Build history of the part. All positions in model axes, mm. Face numbers are marked on the shaded views. A direction names the side the tool comes from. Round coordinates to 2 decimals unless told otherwise and drop trailing zeros. Write each loop counter-clockwise with the first axis right and the second up, starting at its lowest first coordinate (ties: lowest second). Pieces come first, ordered by that corner, then holes.
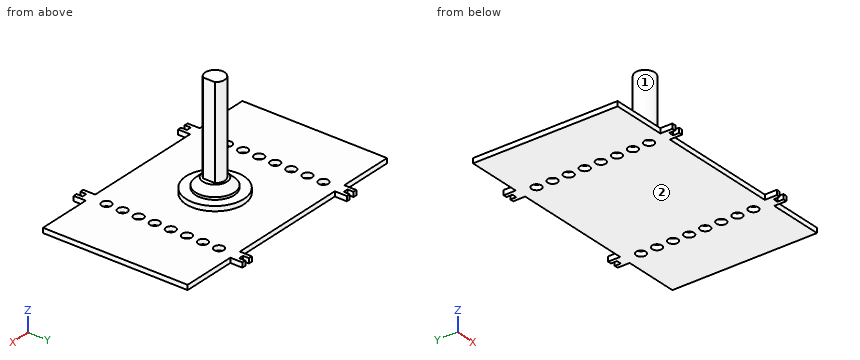
from build123d import *

# Parameters (mm, degrees)
SKETCH_R     = 2
PAD_DEPTH    = 2
SKETCH001_R  = 4
PAD001_DEPTH = 46
SKETCH002_R  = 8
PAD002_DEPTH = 8
SKETCH003_R  = 12
PAD003_DEPTH = 4
POCKET_DEPTH = 38
CHAMFER_SIZE = 3


with BuildPart() as part:
    # Sketch → Pad (new body)
    with BuildSketch(Plane.XY):
        Polygon((105, 0), (105, 60), (82.5, 60), (82.5, 65), (81, 65), (81, 62.5), (80, 62.5), (79, 62.5), (79, 65), (77.5, 65), (77.5, 60), (27.5, 60), (27.5, 65), (26, 65), (26, 62.5), (25, 62.5), (24, 62.5), (24, 65), (22.5, 65), (22.5, 60), (0, 60), (0, 0), (22.5, 0), (22.5, -5), (24, -5), (24, -2.5), (25, -2.5), (26, -2.5), (26, -5), (27.5, -5), (27.5, 0), (77.5, 0), (77.5, -5), (79, -5), (79, -2.5), (80, -2.5), (81, -2.5), (81, -5), (82.5, -5), (82.5, 0), align=None)
        with Locations((25, 46.666667)):
            Circle(SKETCH_R, mode=Mode.SUBTRACT)
        with Locations((25, 40)):
            Circle(SKETCH_R, mode=Mode.SUBTRACT)
        with Locations((25, 33.333333)):
            Circle(SKETCH_R, mode=Mode.SUBTRACT)
        with Locations((25, 26.666667)):
            Circle(SKETCH_R, mode=Mode.SUBTRACT)
        with Locations((25, 20)):
            Circle(SKETCH_R, mode=Mode.SUBTRACT)
        with Locations((25, 13.333333)):
            Circle(SKETCH_R, mode=Mode.SUBTRACT)
        with Locations((25, 6.666667)):
            Circle(SKETCH_R, mode=Mode.SUBTRACT)
        with Locations((80, 6.666667)):
            Circle(SKETCH_R, mode=Mode.SUBTRACT)
        with Locations((80, 13.333333)):
            Circle(SKETCH_R, mode=Mode.SUBTRACT)
        with Locations((80, 20)):
            Circle(SKETCH_R, mode=Mode.SUBTRACT)
        with Locations((80, 26.666667)):
            Circle(SKETCH_R, mode=Mode.SUBTRACT)
        with Locations((80, 33.333333)):
            Circle(SKETCH_R, mode=Mode.SUBTRACT)
        with Locations((80, 46.666667)):
            Circle(SKETCH_R, mode=Mode.SUBTRACT)
        with Locations((80, 40)):
            Circle(SKETCH_R, mode=Mode.SUBTRACT)
        with Locations((25, 53.333333)):
            Circle(SKETCH_R, mode=Mode.SUBTRACT)
        with Locations((80, 53.333333)):
            Circle(SKETCH_R, mode=Mode.SUBTRACT)
    extrude(amount=PAD_DEPTH)

    # Sketch001 → Pad001 (join)
    with BuildSketch(Plane.XY):
        with Locations((52.5, 30)):
            Circle(SKETCH001_R)
    extrude(amount=PAD001_DEPTH)

    # Sketch002 → Pad002 (join)
    with BuildSketch(Plane.XY):
        with Locations((52.5, 30)):
            Circle(SKETCH002_R)
    extrude(amount=PAD002_DEPTH)

    # Sketch003 → Pad003 (join)
    with BuildSketch(Plane.XY):
        with Locations((52.5, 30)):
            Circle(SKETCH003_R)
    extrude(amount=PAD003_DEPTH)

    # Sketch004 → Pocket (cut)
    with BuildSketch(Plane.XY.offset(46)):
        with BuildLine():
            Line((55.622499, 32.5), (55.622499, 27.5))
            ThreePointArc((55.622499, 27.5), (56.5, 30), (55.622499, 32.5))
        make_face()
    extrude(amount=-POCKET_DEPTH, mode=Mode.SUBTRACT)

    # Chamfer
    chamfer_edges = [part.edges().sort_by_distance(p)[0] for p in [
        (44.5, 30, 8),
    ]]
    chamfer(chamfer_edges, length=CHAMFER_SIZE)


solid = part.part
1) Which spindle directions (+Z, -Z, +X, -X, +Y, -Y) get a long thin tool onto all of the face, cutting with end or side? Do the marked faces 1 and 2. Say none if no direction does.
Results:
face 1: +Z
face 2: -Z, +X, -X, +Y, -Y
2) Slice it at B-B (x = 52.5). Write the cut outline in (y, z).
Results:
outline: (0, 0) - (60, 0) - (60, 2) - (42, 2) - (42, 4) - (38, 4) - (38, 5) - (35, 8) - (34, 8) - (34, 46) - (26, 46) - (26, 8) - (25, 8) - (22, 5) - (22, 4) - (18, 4) - (18, 2) - (0, 2) - close
3) Pin check, flat tips, straight feed: pin 1 Ø4.5 at (x, y) = (80, 26.67) entering from +Z; pin 2 Ø0.6 at (x, z) = (90, 1) entering from -Y; pin 3 Ø3 at (x, y) = (25, 20) entering from -Z; pin 4 Ø8 at (y, z) = (27, 21) entering from -X. Stop position of each tip, or through.
Results:
pin 1: stops at z = 2
pin 2: stops at y = 0
pin 3: passes through
pin 4: stops at x = 48.5
4) Slice it at A-A (y = 20). Write the cut outline in (x, z).
Results:
outline: (0, 0) - (23, 0) - (23, 2) - (0, 2) - close; (27, 0) - (78, 0) - (78, 2) - (59.13, 2) - (59.13, 4) - (45.87, 4) - (45.87, 2) - (27, 2) - close; (82, 0) - (105, 0) - (105, 2) - (82, 2) - close
5) Slice it at C-C (y = 30). Write the cut outline in (x, z).
Results:
outline: (0, 0) - (105, 0) - (105, 2) - (64.5, 2) - (64.5, 4) - (60.5, 4) - (60.5, 5) - (57.5, 8) - (55.62, 8) - (55.62, 46) - (48.5, 46) - (48.5, 8) - (47.5, 8) - (44.5, 5) - (44.5, 4) - (40.5, 4) - (40.5, 2) - (0, 2) - close
6) Wall check: L1, parallel to Z at x = 29, y = 20; L2, parallel to X at y = 29, z = 31; L3, parallel to Y at x = 54, z = 10. Give the ranges that are in metal, low to high.
Results:
L1: z = 0 to 2
L2: x = 48.63 to 55.62
L3: y = 26.29 to 33.71
7) Slice it at D-D (z = 35.5). Write the cut outline in (x, y).
Results:
outline: (55.62, 27.5) - (55.62, 32.5) arc R4 ccw (long way) to start
